```python
from build123d import *

# Parameters (mm, degrees)
F0_W      = 5.4
F0_H      = 40
F1_DEPTH  = 5.5
F2_W      = 1.5
F2_H      = 6.1
F3_DEPTH  = 5.501
F4_W      = 1.5
F4_H      = 6.1
F5_DEPTH  = 25
F6_W      = 1.5
F6_H      = 6.1
F7_DEPTH  = 5.501
F8_W      = 1.5
F8_H      = 6.1
F9_DEPTH  = 5.501
F10_R     = 2.75
F11_R     = 2.74999
F12_R     = 2.75
F13_R     = 2.74999
F14_W     = 2.3
F14_H     = 24.25
F15_DEPTH = 2.701
F16_DEPTH = 2.701
F17_R     = 1.15
F18_R     = 1.14999
F19_R     = 1.15
F20_R     = 1.14999
F21_R     = 0.75
F22_DEPTH = 3.901
F23_R     = 0.75
F24_DEPTH = 3.901


# Not quite as in the source:
# - a fillet or chamfer is up to 0.001 mm smaller than in the source, because OpenCascade refuses the exact size


with BuildPart() as f1:
    # F0 (on Front) → F1 (new body)
    with BuildSketch(Plane.XZ):
        Rectangle(F0_W, F0_H)
    extrude(amount=F1_DEPTH)

    # F2 (on face) → F3 (cut, through all)
    with BuildSketch(Plane.XZ.offset(5.5)):
        with Locations((-1.95, 16.95)):
            Rectangle(F2_W, F2_H)
    extrude(amount=-F3_DEPTH, mode=Mode.SUBTRACT)

    # F4 (on face) → F5 (cut)
    with BuildSketch(Plane.XZ.offset(5.5)):
        with Locations((1.95, 16.95)):
            Rectangle(F4_W, F4_H)
    extrude(amount=-F5_DEPTH, mode=Mode.SUBTRACT)

    # F6 (on face) → F7 (cut, through all)
    with BuildSketch(Plane.XZ.offset(5.5)):
        with Locations((-1.95, -16.95)):
            Rectangle(F6_W, F6_H)
    extrude(amount=-F7_DEPTH, mode=Mode.SUBTRACT)

    # F8 (on face) → F9 (cut, through all)
    with BuildSketch(Plane.XZ.offset(5.5)):
        with Locations((1.95, -16.95)):
            Rectangle(F8_W, F8_H)
    extrude(amount=-F9_DEPTH, mode=Mode.SUBTRACT)

    # F10
    f10_edges = [f1.edges().sort_by_distance(p)[0] for p in [
        (0, -5.5, 20),
    ]]
    fillet(f10_edges, radius=F10_R)

    # F11 (radius 2.75 in the source; OpenCascade refuses exactly that, so slightly less here)
    f11_edges = [f1.edges().sort_by_distance(p)[0] for p in [
        (0, 0, 20),
    ]]
    fillet(f11_edges, radius=F11_R)

    # F12
    f12_edges = [f1.edges().sort_by_distance(p)[0] for p in [
        (0, 0, -20),
    ]]
    fillet(f12_edges, radius=F12_R)

    # F13 (radius 2.75 in the source; OpenCascade refuses exactly that, so slightly less here)
    f13_edges = [f1.edges().sort_by_distance(p)[0] for p in [
        (0, -5.5, -20),
    ]]
    fillet(f13_edges, radius=F13_R)

    # F14 (on Right) → F15 (cut, through all)
    with BuildSketch(Plane.YZ):
        with Locations((-2.75, 0)):
            Rectangle(F14_W, F14_H)
    extrude(amount=-F15_DEPTH, mode=Mode.SUBTRACT)

    # F14 (on Right) → F16 (cut, through all)
    with BuildSketch(Plane.YZ):
        with Locations((-2.75, 0)):
            Rectangle(F14_W, F14_H)
    extrude(amount=F16_DEPTH, mode=Mode.SUBTRACT)

    # F17
    f17_edges = [f1.edges().sort_by_distance(p)[0] for p in [
        (0, -3.9, 12.125),
    ]]
    fillet(f17_edges, radius=F17_R)

    # F18 (radius 1.15 in the source; OpenCascade refuses exactly that, so slightly less here)
    f18_edges = [f1.edges().sort_by_distance(p)[0] for p in [
        (0, -1.6, 12.125),
    ]]
    fillet(f18_edges, radius=F18_R)

    # F19
    f19_edges = [f1.edges().sort_by_distance(p)[0] for p in [
        (0, -3.9, -12.125),
    ]]
    fillet(f19_edges, radius=F19_R)

    # F20 (radius 1.15 in the source; OpenCascade refuses exactly that, so slightly less here)
    f20_edges = [f1.edges().sort_by_distance(p)[0] for p in [
        (0, -1.6, -12.125),
    ]]
    fillet(f20_edges, radius=F20_R)

    # F21 (on face) → F22 (cut, through all)
    with BuildSketch(Plane.YZ.offset(1.2)):
        with Locations((-2.75, 17.25)):
            Circle(F21_R)
    extrude(amount=-F22_DEPTH, mode=Mode.SUBTRACT)

    # F23 (on face) → F24 (cut, through all)
    with BuildSketch(Plane.YZ.offset(1.2)):
        with Locations((-2.75, -17.25)):
            Circle(F23_R)
    extrude(amount=-F24_DEPTH, mode=Mode.SUBTRACT)


solid = f1.part
```
Input: part model. Units: mm. Frame: model coordinates. A direction names the side the tool comes from. Give positions to 0.01 mm unless a question says otherwise; leave off trailing zeros. Order: outer loops, then holes, each group sorted by start corner. A loop starts at its lowest first (then second) coordinate and runs counter-clockwise, first axis right, second up.
1. Pin query (flat end, axial travel): pin 1 Ø0.5 at (x, y) = (-2.5, -1.5) entering from +Z; pin 2 Ø1.2 at (x, y) = (2, -2.5) entering from -Z; pin 3 Ø1.7 at (y, z) = (-2.75, -17.25) entering from +X. Return the tip coordinate at first contact, or that it passes through.
Computed:
pin 1: stops at z = 13.9
pin 2: stops at z = -13.9
pin 3: stops at x = 1.2
2. Draft query along Y for faces 4 (the face through (0.04, -1.95, 11.8)), 5 (the face through (0.02, -0.78, -19.17)), 6 (the face through (0.02, -4.72, 19.17)), 7 (the face through (1.2, -3, -16)). Return one class per face: released by +Y, released by -Y, zero draft, split by the parting line, or undercut.
Computed:
face 4: undercut
face 5: released by +Y
face 6: released by -Y
face 7: zero draft
3. Cut plane A-A (z = 4). Return loops of the section in (x, y), and give its area (3 significant figures).
Computed:
outline: (-2.7, -5.5) - (2.7, -5.5) - (2.7, -3.9) - (-2.7, -3.9) - close; (-2.7, -1.6) - (2.7, -1.6) - (2.7, 0) - (-2.7, 0) - close
area: 17.3 mm2
4. Line query: probe 1 along Y at (x, z) = (-1.7, -7.5); probe 2 along Z at (x, y) = (1.9, -3.4); probe 3 along Z at (x, y) = (-1.75, -4.35). Output: solid intervals per line, ascending.
Computed:
probe 1: y = -5.5 to -3.9, -1.6 to 0
probe 2: z = -13.9 to -11.92, 11.92 to 13.9
probe 3: z = -13.9 to 13.9
5. Cut plane D-D (y = -4.45). Return loops of the section in (x, z).
Computed:
outline: (-2.7, -13.9) - (-1.2, -13.9) - (-1.2, -19.41) - (1.2, -19.41) - (1.2, -13.9) - (2.7, -13.9) - (2.7, 13.9) - (1.2, 13.9) - (1.2, 19.41) - (-1.2, 19.41) - (-1.2, 13.9) - (-2.7, 13.9) - close
6. Set-up query: faces 1 (the face through (-0.04, -3.57, 11.78)), 2 (the face through (2, -3, 13.9)), 3 (the face through (-2, -3, -13.9)). Return all of +Z, -Z, +X, -X, +Y, -Y with unobstructed straight access to the full face (end or side cutting, diameter ignored); none if empty.
Computed:
face 1: +X, -X
face 2: +Z, +X, +Y, -Y
face 3: -Z, -X, +Y, -Y
7. Cut plane B-B (x = -0.75). State how many separate pieces and enclosed holes the cut face has, and give its area (3 significant figures).
Computed:
separate pieces: 1
enclosed holes: 3
area: 155 mm2
8. Cut plane C-C (y = -1.2). Return loops of the section in (x, z), and give its area (3 significant figures).
Computed:
outline: (-2.7, -13.9) - (-1.2, -13.9) - (-1.2, -19.52) - (1.2, -19.52) - (1.2, -13.9) - (2.7, -13.9) - (2.7, 13.9) - (1.2, 13.9) - (1.2, 19.52) - (-1.2, 19.52) - (-1.2, 13.9) - (-2.7, 13.9) - close
area: 177 mm2
